Read the model definition and answer for the solid it produces. Units are mm, in the model's axes. A direction names the side the tool comes from. Round coordinates to 2 decimals unless told otherwise and drop trailing zeros. Loops run counter-clockwise (first coordinate to the right, second up) from the corner with the lowest first, then second, coordinate; pieces in that order, holes last. Notation, with made-up numbers: M 28.25,29.5 L 40.25,29.5 A15 ccw 40.25,37.5 Z; hole C 87.5,-37 d2. An arc over 180 degrees is marked long. Write each question's results on one line, items separated by ' | '.
```python
from build123d import *

# Parameters (mm, degrees)
F_01_START                                     = -3.6
S01_BALL_AND_MISALIGNMENT_SPACER_LAND_R        = 1.83
S01_BALL_AND_MISALIGNMENT_SPACER_LAND_R_2      = 1.52
F_01_BALL_AND_MISALIGNMENT_SPACER_LAND_1_DEPTH = 1.6
F_02_START                                     = -2
S02_BALL_AND_MISALIGNMENT_SPACER_LAND_R        = 2
S02_BALL_AND_MISALIGNMENT_SPACER_LAND_R_2      = 1.52
F_02_BALL_AND_MISALIGNMENT_SPACER_LAND_2_DEPTH = 0.4
F_03_START                                     = -1.6
S03_BALL_AND_MISALIGNMENT_SPACER_LAND_R        = 2.31
S03_BALL_AND_MISALIGNMENT_SPACER_LAND_R_2      = 1.52
F_03_BALL_AND_MISALIGNMENT_SPACER_LAND_3_DEPTH = 0.4
F_04_START                                     = -1.2
S04_BALL_AND_MISALIGNMENT_SPACER_LAND_R        = 2.55
S04_BALL_AND_MISALIGNMENT_SPACER_LAND_R_2      = 1.52
F_04_BALL_AND_MISALIGNMENT_SPACER_LAND_4_DEPTH = 0.6
F_05_START                                     = -0.6
S05_BALL_AND_MISALIGNMENT_SPACER_LAND_R        = 2.76
S05_BALL_AND_MISALIGNMENT_SPACER_LAND_R_2      = 1.52
F_05_BALL_AND_MISALIGNMENT_SPACER_LAND_5_DEPTH = 1.2
F_06_START                                     = 0.6
S06_BALL_AND_MISALIGNMENT_SPACER_LAND_R        = 2.55
S06_BALL_AND_MISALIGNMENT_SPACER_LAND_R_2      = 1.52
F_06_BALL_AND_MISALIGNMENT_SPACER_LAND_6_DEPTH = 0.6
F_07_START                                     = 1.2
S07_BALL_AND_MISALIGNMENT_SPACER_LAND_R        = 2.31
S07_BALL_AND_MISALIGNMENT_SPACER_LAND_R_2      = 1.52
F_07_BALL_AND_MISALIGNMENT_SPACER_LAND_7_DEPTH = 0.4
F_08_START                                     = 1.6
S08_BALL_AND_MISALIGNMENT_SPACER_LAND_R        = 2
S08_BALL_AND_MISALIGNMENT_SPACER_LAND_R_2      = 1.52
F_08_BALL_AND_MISALIGNMENT_SPACER_LAND_8_DEPTH = 0.4
F_09_START                                     = 2
S09_BALL_AND_MISALIGNMENT_SPACER_LAND_R        = 1.83
S09_BALL_AND_MISALIGNMENT_SPACER_LAND_R_2      = 1.52
F_09_BALL_AND_MISALIGNMENT_SPACER_LAND_9_DEPTH = 1.6


with BuildPart() as part:
    # S01 - Ball and misalignment spacer land 1 → 01 - Ball and misalignment spacer land 1 (new body)
    with BuildSketch(Plane.XY.offset(F_01_START)):
        Circle(S01_BALL_AND_MISALIGNMENT_SPACER_LAND_R)
        Circle(S01_BALL_AND_MISALIGNMENT_SPACER_LAND_R_2, mode=Mode.SUBTRACT)
    extrude(amount=F_01_BALL_AND_MISALIGNMENT_SPACER_LAND_1_DEPTH)

    # S02 - Ball and misalignment spacer land 2 → 02 - Ball and misalignment spacer land 2 (add)
    with BuildSketch(Plane.XY.offset(F_02_START)):
        Circle(S02_BALL_AND_MISALIGNMENT_SPACER_LAND_R)
        Circle(S02_BALL_AND_MISALIGNMENT_SPACER_LAND_R_2, mode=Mode.SUBTRACT)
    extrude(amount=F_02_BALL_AND_MISALIGNMENT_SPACER_LAND_2_DEPTH)

    # S03 - Ball and misalignment spacer land 3 → 03 - Ball and misalignment spacer land 3 (add)
    with BuildSketch(Plane.XY.offset(F_03_START)):
        Circle(S03_BALL_AND_MISALIGNMENT_SPACER_LAND_R)
        Circle(S03_BALL_AND_MISALIGNMENT_SPACER_LAND_R_2, mode=Mode.SUBTRACT)
    extrude(amount=F_03_BALL_AND_MISALIGNMENT_SPACER_LAND_3_DEPTH)

    # S04 - Ball and misalignment spacer land 4 → 04 - Ball and misalignment spacer land 4 (add)
    with BuildSketch(Plane.XY.offset(F_04_START)):
        Circle(S04_BALL_AND_MISALIGNMENT_SPACER_LAND_R)
        Circle(S04_BALL_AND_MISALIGNMENT_SPACER_LAND_R_2, mode=Mode.SUBTRACT)
    extrude(amount=F_04_BALL_AND_MISALIGNMENT_SPACER_LAND_4_DEPTH)

    # S05 - Ball and misalignment spacer land 5 → 05 - Ball and misalignment spacer land 5 (add)
    with BuildSketch(Plane.XY.offset(F_05_START)):
        Circle(S05_BALL_AND_MISALIGNMENT_SPACER_LAND_R)
        Circle(S05_BALL_AND_MISALIGNMENT_SPACER_LAND_R_2, mode=Mode.SUBTRACT)
    extrude(amount=F_05_BALL_AND_MISALIGNMENT_SPACER_LAND_5_DEPTH)

    # S06 - Ball and misalignment spacer land 6 → 06 - Ball and misalignment spacer land 6 (add)
    with BuildSketch(Plane.XY.offset(F_06_START)):
        Circle(S06_BALL_AND_MISALIGNMENT_SPACER_LAND_R)
        Circle(S06_BALL_AND_MISALIGNMENT_SPACER_LAND_R_2, mode=Mode.SUBTRACT)
    extrude(amount=F_06_BALL_AND_MISALIGNMENT_SPACER_LAND_6_DEPTH)

    # S07 - Ball and misalignment spacer land 7 → 07 - Ball and misalignment spacer land 7 (add)
    with BuildSketch(Plane.XY.offset(F_07_START)):
        Circle(S07_BALL_AND_MISALIGNMENT_SPACER_LAND_R)
        Circle(S07_BALL_AND_MISALIGNMENT_SPACER_LAND_R_2, mode=Mode.SUBTRACT)
    extrude(amount=F_07_BALL_AND_MISALIGNMENT_SPACER_LAND_7_DEPTH)

    # S08 - Ball and misalignment spacer land 8 → 08 - Ball and misalignment spacer land 8 (add)
    with BuildSketch(Plane.XY.offset(F_08_START)):
        Circle(S08_BALL_AND_MISALIGNMENT_SPACER_LAND_R)
        Circle(S08_BALL_AND_MISALIGNMENT_SPACER_LAND_R_2, mode=Mode.SUBTRACT)
    extrude(amount=F_08_BALL_AND_MISALIGNMENT_SPACER_LAND_8_DEPTH)

    # S09 - Ball and misalignment spacer land 9 → 09 - Ball and misalignment spacer land 9 (add)
    with BuildSketch(Plane.XY.offset(F_09_START)):
        Circle(S09_BALL_AND_MISALIGNMENT_SPACER_LAND_R)
        Circle(S09_BALL_AND_MISALIGNMENT_SPACER_LAND_R_2, mode=Mode.SUBTRACT)
    extrude(amount=F_09_BALL_AND_MISALIGNMENT_SPACER_LAND_9_DEPTH)


solid = part.part
```
1. Find section B-B, the plane z = 2.75. Give the vertices of the cut face in (x, y).
Completed:
outline: C 0,0 d3.66; hole C 0,0 d3.04
2. Which of the six approach directions +Z, -Z, +X, -X, +Y, -Y give full straight-line access (tool end or side, diameter ignored) to faces 3 (the face through (-0.598, -2.694, -0.008)), 4 (the face through (1.18, -2.26, -0.9)), 5 (the face through (-0.434, -1.952, 1.797))?
Completed:
face 3: +Z, -Z | face 4: -Z | face 5: +Z
3. Determine the mould class of faces 1 (the face through (-1.452, -1.114, -2.811)), 2 (the face through (1.45, 0.46, -0.05)) for opening direction X: released by +X, released by -X, zero draft, split by the parting line, or undercut.
Completed:
face 1: split by the parting line | face 2: undercut
4. Find section A-A, the plane z = -0.25. Give the vertices of the cut face in (x, y), then the cut area to 3 significant figures.
Completed:
outline: C 0,0 d5.52; hole C 0,0 d3.04 | area: 16.7 mm2
5. Given P1, Ø3, axis at x = -1, z = 2.5, coming from the -Y side; P2, Ø3, axis at x = 1.5, z = -1.5, coming from the -Y side; P3, Ø1.4, axis at x = 0, y = -0.5, coming from the -Z side; P4, Ø1, axis at y = -1, z = -1, coming from the +X side, each flat-ended and moving along its own axis, determine where each tip first touches the part or whether it passes through.
Completed:
P1: stops at y = -2.54 | P2: stops at y = -2.74 | P3: passes through | P4: stops at x = 2.67
6. Find the intervals of material crossed by L1, parallel to Y at x = 0, z = 0.5; L2, parallel to Y at x = 0, z = 1; L3, parallel to X at y = -0.6, z = 0, in increasing order.
Completed:
L1: y = -2.76 to -1.52, 1.52 to 2.76 | L2: y = -2.55 to -1.52, 1.52 to 2.55 | L3: x = -2.69 to -1.4, 1.4 to 2.69
